Part model, mm, in its own coordinate system. Face numbers are marked on the shaded views. Round coordinates to 2 decimals unless told otherwise and drop trailing zeros. Write each loop counter-clockwise with the first axis right and the second up, starting at its lowest first coordinate (ties: lowest second). Pieces come first, ordered by that corner, then holes. Notation, with made-up numbers: (29, 11.5) -> (86, 11.5) arc R12 ccw to (86, 18.5) -> close; hole circle Ø9 at (88.5, 48). An arc over 180 degrees is marked (long way). Return JSON: item names as keys, results as strings. Group by question number.
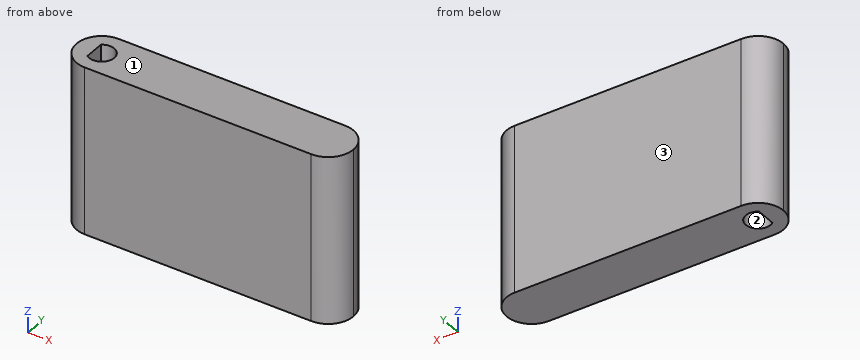
```python
from build123d import *

# Parameters (mm, degrees)
SKETCH1_W           = 66
SKETCH1_H           = 12
SKETCH1_R           = 2.98
BOSS_EXTRUDE1_DEPTH = 20
FILLET2_R           = 6
BOSS_EXTRUDE2_DEPTH = 40


with BuildPart() as part:
    # Sketch1 → Boss-Extrude1 (new, symmetric)
    with BuildSketch(Plane.XY):
        with Locations((27, 0)):
            Rectangle(SKETCH1_W, SKETCH1_H)
        Circle(SKETCH1_R, mode=Mode.SUBTRACT)
    extrude(amount=BOSS_EXTRUDE1_DEPTH, both=True)

    # Fillet2
    fillet2_edges = [part.edges().sort_by_distance(p)[0] for p in [
        (60, -6, 0),
        (60, 6, 0),
        (-6, -6, 0),
        (-6, 6, 0),
    ]]
    fillet(fillet2_edges, radius=FILLET2_R - 0.0001)  # a hair under: the kernel refuses the full size

    # Sketch2 → Boss-Extrude2 (add)
    with BuildSketch(Plane(origin=(0, 0, -20), x_dir=(-1, 0, 0), z_dir=(0, 0, -1))):
        with BuildLine():
            Line((1.8, -2.374952631), (1.8, 2.374952631))
            ThreePointArc((1.8, 2.374952631), (2.98, 0), (1.8, -2.374952631))
        make_face()
    extrude(amount=-BOSS_EXTRUDE2_DEPTH)


solid = part.part
```
Item 1: Flat gauge pins, fed straight in: P1, Ø4, axis at y = 4.5, z = -1.5, coming from the -X side; P2, Ø1.5, axis at y = -3.5, z = -13, coming from the -X side. Where does each tip first touch, or does it go through?
Item 2: Cut at B-B (y = -4). Write the cut outline in (x, z).
Item 3: Wall check: L1, parallel to Y at x = 0, z = 11; L2, parallel to X at y = 0, z = 7; L3, parallel to X at y = 1.75, z = 2. Give the ranges that are in metal, low to high.
Item 4: Two-plate mould, pull along Y, no slides. Class the marked faces 1, 2 and 3: released by +Y, released by -Y, zero draft, split by the parting line, or undercut.
Checks:
{
 "1": {"P1": "stops at x = -5.45", "P2": "stops at x = -5.33"},
 "2": {"outline": "(-4.47, -20) -> (58.47, -20) -> (58.47, 20) -> (-4.47, 20) -> close"},
 "3": {"L1": "y = -6 to -2.98, 2.98 to 6", "L2": "x = -6 to -1.8, 2.98 to 60", "L3": "x = -5.74 to -1.8, 2.41 to 59.74"},
 "4": {"face 1": "zero draft", "face 2": "undercut", "face 3": "released by +Y"}
}
